Could you check a few things on this model? Use its own coordinates, in mm. A direction names the side the tool comes from. Coordinates: 2 decimals unless noted, no trailing zeros. Order: outer loops, then holes, each group sorted by start corner. A loop starts at its lowest first (then second) coordinate and runs counter-clockwise, first axis right, second up. Notation, with made-up numbers: (42.25, 60) - (101.25, 60) arc R35 cw to (101.25, 93) - close; hole circle Ø7 at (-15.75, -9.75). An arc over 180 degrees is marked (long way). One line per item, written item: value. Start each with the question number.
Autodesk Inventor part; units mm, degrees
ref_plane "YZ Plane" through (0, 0, 0) normal (1, 0, 0) x (0, 1, 0)
ref_plane "XY Plane" through (0, 0, 0) normal (0, 0, 1) x (1, 0, 0)
sketch "Sketch1" plane through (0, 0, 0) normal (0, 1, 0) x (-1, 0, 0)
  line L0 (-80, 80) -> (80, 80)
  line L1 (80, 80) -> (80, -80)
  line L2 (80, -80) -> (-80, -80)
  line L3 (-80, -80) -> (-80, 80)
  line L4 (-80, 80) -> (80, -80) construction
  line L5 (80, 80) -> (-80, -80) construction
  point P0 (0, 0)
  dimension "d0" = 160
  dimension "d1" = 160
ref_plane "Work Plane3" through (0, 180, 0) normal (0, 1, 0) x (-1, 0, 0)
sketch "Sketch7" plane through (0, 180, 0) normal (0, 1, 0) x (-1, 0, 0)
  point P0 (0, 0)
  point P1 (0, 0)
loft "Loft2" add profiles "Sketch1" section 2 point at (0, 180, 0)
shell "Shell2" thickness 2 removed faces 1 at (26.6667, 0, 26.6667)
properties part number "pyramid"
Q1. I want a section at B-B on z = -63. Please give me the cut outline in (x, y).
Q2. If I drill on L1, parallel to Z at x = -9, y = 51.5; L2, parallel to X at y = 69, z = -23.5; L3, parallel to X at y = 73.5, z = 8.5, over which ranges is the centre line in solid material (lowest first)?
Q3. I want a section at C-C on x = 42.5. Please give me the cut outline in (y, z) (3 decimals).
Q4. We'd pull the mould along Z, two halves only. Please class faces 3 (the flat face through (1.12, 71.26, -48.33)), 4 (the flat face through (1.089, 69.31, -47.007)), 5 (the flat face through (-48.33, 71.26, -1.12)): +Z half, -Z half, draft (parallel to the pull), parting line (faces both ways), or undercut.
Q5. I want a section at D-D on y = 30. Please give me the cut outline in (x, z), then the cut area to 3 significant figures.
Q6. I want a section at A-A on y = 78. Please give me the cut outline in (x, z).
Q7. Which directions (+Z, -Z, +X, -X, +Y, -Y) give clear straight access to the entire face, cutting with the end or side of a thin tool? Please do faces 1 (the flat face through (47.007, 69.31, 1.089)), 2 (the flat face through (48.33, 71.26, 1.12)).
Q8. I'm going to push flat-ended pins straight in: pin 1 (5 mm diameter, centred on x = 36, z = 21, fed in from +Y) (3 decimals); pin 2 (4 mm diameter, centred on x = 21.5, z = -13.5, fed in from +Y) (3 decimals); pin 3 (6 mm diameter, centred on x = -46.5, y = 44.5, fed in from +Z). Where does each tip first touch, or does it pass through?
Values follow:
1. outline: (-80, 0) - (-77.81, 0) - (-63, 33.33) - (63, 33.33) - (77.81, 0) - (80, 0) - (63, 38.25) - (-63, 38.25) - close
2. L1: z = -57.11 to -54.92, 54.92 to 57.11
2. L2: x = -49.33 to -47.14, 47.14 to 49.33
2. L3: x = -47.33 to -45.14, 45.14 to 47.33
3. outline: (0, -80) - (84.375, -42.5) - (84.375, 42.5) - (0, 80) - (0, 77.811) - (79.451, 42.5) - (79.451, -42.5) - (0, -77.811) - close
4. face 3: -Z half
4. face 4: undercut
4. face 5: draft
5. outline: (-66.67, -66.67) - (66.67, -66.67) - (66.67, 66.67) - (-66.67, 66.67) - close; hole (-64.48, -64.48) - (64.48, -64.48) - (64.48, 64.48) - (-64.48, 64.48) - close
5. area: 1,150 mm^2
6. outline: (-45.33, -45.33) - (45.33, -45.33) - (45.33, 45.33) - (-45.33, 45.33) - close; hole (-43.14, -43.14) - (43.14, -43.14) - (43.14, 43.14) - (-43.14, 43.14) - close
7. face 1: -Y
7. face 2: +Z, -Z, +X, +Y
8. pin 1: stops at y = 104.625
8. pin 2: stops at y = 136.125
8. pin 3: stops at z = 61.56
